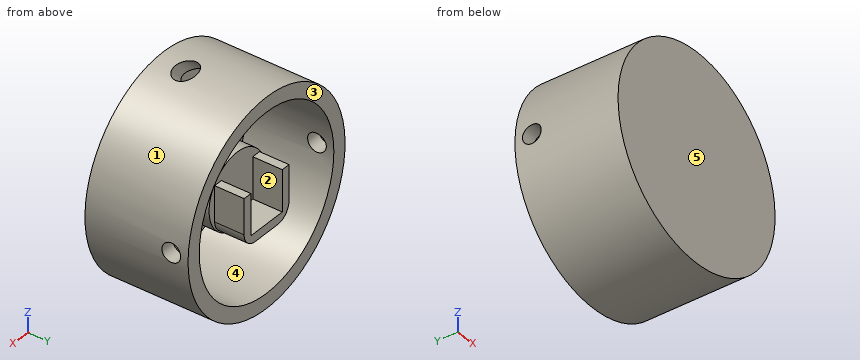
```python
from build123d import *

# Parameters (mm, degrees)
SKETCH1_R           = 35
BOSS_EXTRUDE1_DEPTH = 35
SKETCH3_R           = 30
CUT_EXTRUDE1_DEPTH  = 30
SKETCH4_R           = 12.5
BOSS_EXTRUDE2_DEPTH = 20
SKETCH5_R           = 3.6
CUT_EXTRUDE2_DEPTH  = 20
BOSS_EXTRUDE3_DEPTH = 10
SKETCH8_R           = 3.175
CUT_EXTRUDE4_DEPTH  = 67.895440973
SKETCH10_R          = 3.175
CUT_EXTRUDE5_DEPTH  = 67.895440995


with BuildPart() as part:
    # Sketch1 → Boss-Extrude1 (new body)
    with BuildSketch(Plane(origin=(0, 0, 0), x_dir=(1, 0, 0), z_dir=(0, 1, 0))):
        with Locations(Location((0, 0, 0), (0, 0, 270))):
            Circle(SKETCH1_R)
    extrude(amount=BOSS_EXTRUDE1_DEPTH)

    # Sketch3 → Cut-Extrude1 (cut)
    with BuildSketch(Plane(origin=(0, 35, 0), x_dir=(1, 0, 0), z_dir=(0, 1, 0))):
        with Locations(Location((0, 0, 0), (0, 0, 270))):
            Circle(SKETCH3_R)
    extrude(amount=-CUT_EXTRUDE1_DEPTH, mode=Mode.SUBTRACT)

    # Sketch4 → Boss-Extrude2 (add)
    with BuildSketch(Plane(origin=(0, 5, 0), x_dir=(1, 0, 0), z_dir=(0, 1, 0))):
        with Locations(Location((0, 0, 0), (0, 0, 270))):
            Circle(SKETCH4_R)
    extrude(amount=BOSS_EXTRUDE2_DEPTH)

    # Sketch5 → Cut-Extrude2 (cut)
    with BuildSketch(Plane(origin=(24.748737342, 0, 24.748737342), x_dir=(0, -1, 0), z_dir=(0.7071067811865488, 0, 0.7071067811865464))):
        with Locations(Location((-10, -22.260066462, 0), (0, 0, 90))):
            Circle(SKETCH5_R)
    extrude(amount=-CUT_EXTRUDE2_DEPTH, mode=Mode.SUBTRACT)

    # Sketch6 → Boss-Extrude3 (add)
    with BuildSketch(Plane(origin=(0, 25, 0), x_dir=(1, 0, 0), z_dir=(0, 1, 0))):
        with BuildLine():
            Line((-10, -7), (-10, 5))
            ThreePointArc((-10, 5), (-8.535533906, 8.535533906), (-5, 10))
            Line((-5, 10), (5, 10))
            ThreePointArc((5, 10), (8.535533906, 8.535533906), (10, 5))
            Line((10, 5), (10, -7))
            Line((10, -7), (7, -7))
            Line((7, -7), (7, 7))
            Line((7, 7), (-7, 7))
            Line((-7, 7), (-7, -7))
            Line((-7, -7), (-10, -7))
        make_face()
    extrude(amount=BOSS_EXTRUDE3_DEPTH)

    # Sketch8 → Cut-Extrude4 (cut, through all)
    with BuildSketch(Plane(origin=(10, 0, 0), x_dir=(0, 0, -1), z_dir=(1, 0, 0))):
        with Locations(Location((-0.65, 29.285, 0), (0, 0, 180))):
            Circle(SKETCH8_R)
    extrude(amount=CUT_EXTRUDE4_DEPTH, mode=Mode.SUBTRACT)

    # Sketch10 → Cut-Extrude5 (cut, through all)
    with BuildSketch(Plane.ZY.offset(10)):
        with Locations((0.65, 29.285)):
            Circle(SKETCH10_R)
    extrude(amount=CUT_EXTRUDE5_DEPTH, mode=Mode.SUBTRACT)


solid = part.part
```
Geometry check sheet. Reference: the model listing, model coordinates, mm. Face numbers are marked on the shaded views. A direction names the side the tool comes from. Coordinates: 2 decimals unless noted, no trailing zeros. Order: outer loops, then holes, each group sorted by start corner. A loop starts at its lowest first (then second) coordinate and runs counter-clockwise, first axis right, second up.
Item 1: Section check C-C (y = 11). Enter the section's corners in (x, z), plus the area to 3 significant figures.
Item 2: Scan lines: line 1 along X through (y, z) = (12, 0); line 2 along X through (y, z) = (12, -1.5); line 3 along Y through (x, z) = (-30.8, 0.65). Record each from-to range of solid material in increasing order.
Item 3: Mould release check, pull along Z, two halves, no side actions. Record for the marked faces 1, 2 and 3: released by +Z, released by -Z, zero draft, split by the parting line, or undercut.
Item 4: Section check D-D (z = 23). Enter the section's corners in (x, y), plus the area to 3 significant figures.
Item 5: Depth check by flat-ended pin: pin 1 (3 mm diameter, centred on y = 32, z = 2, fed in from -X); pin 2 (3.5 mm diameter, centred on x = 9, y = 28, fed in from +Z); pin 3 (12 mm diameter, centred on x = -22.5, y = 10.5, fed in from -Z). Enter the tip coordinate at first touch or a pass-through.
Item 6: Section check A-A (z = -1). Enter the section's corners in (x, y), plus the area to 3 significant figures.
Item 7: Section check B-B (x = 9). Enter the section's corners in (y, z), plus the area to 3 significant figures.
Item 8: Tool access check on the marked faces 4 and 5. Record the directions out of +Z, -Z, +X, -X, +Y, -Y that give a thin tool (end or side, any length) a straight path to the whole face; none if there is none.
Check sheet entries:
1. outline: circle Ø25 at (0, 0); (-7.26, 29.11) - (-1.4, 34.97) arc R35 ccw (long way) to (7.58, 34.17) - (3.24, 29.83) arc R30 cw (long way) to start
1. area: 1,460 mm2
2. line 1: x = -35 to -30, -12.5 to 12.5, 30 to 35
2. line 2: x = -34.97 to -29.96, -12.41 to 12.41, 29.96 to 34.97
2. line 3: y = 0 to 26.11, 32.46 to 35
3. face 1: split by the parting line
3. face 2: undercut
3. face 3: zero draft
4. outline: (-26.38, 0) - (26.38, 0) - (26.38, 35) - (19.26, 35) - (19.26, 5) - (-19.26, 5) - (-19.26, 35) - (-26.38, 35) - close
4. area: 691 mm2
5. pin 1: stops at x = -35
5. pin 2: stops at z = 34.24
5. pin 3: stops at z = -30.87
6. outline: (-34.99, 0) - (34.99, 0) - (34.99, 26.57) - (29.98, 26.57) - (29.98, 5) - (12.46, 5) - (12.46, 25) - (10, 25) - (10, 35) - (7, 35) - (7, 25) - (-7, 25) - (-7, 35) - (-10, 35) - (-10, 25) - (-12.46, 25) - (-12.46, 5) - (-29.98, 5) - (-29.98, 26.57) - (-34.99, 26.57) - close; (-34.99, 32) - (-29.98, 32) - (-29.98, 35) - (-34.99, 35) - close; (29.98, 32) - (34.99, 32) - (34.99, 35) - (29.98, 35) - close
6. area: 1,150 mm2
7. outline: (0, -33.82) - (35, -33.82) - (35, -28.62) - (5, -28.62) - (5, -8.67) - (25, -8.67) - (25, -8) - (35, -8) - (35, 7) - (25, 7) - (25, 8.67) - (5, 8.67) - (5, 28.62) - (35, 28.62) - (35, 33.82) - (0, 33.82) - close
7. area: 1,150 mm2
8. face 4: +Y
8. face 5: +Z, -Z, +X, -X, -Y
